```python
from build123d import *

# Parameters (mm, degrees)
F0_W     = 100.119468
F0_H     = 86.142674
F1_DEPTH = 50.8
F2_R     = 25.4
F4_D     = 25.4


with BuildPart() as f1:
    # F0 (on Front) → F1 (new body)
    with BuildSketch(Plane.XZ):
        with Locations((1.568822, 9.270322)):
            Rectangle(F0_W, F0_H)
    extrude(amount=F1_DEPTH)

    # F2
    f2_edges = [f1.edges().sort_by_distance(p)[0] for p in [
        (51.628556, -25.4, 52.341659),
        (-48.490912, -25.4, 52.341659),
        (-48.490912, -25.4, -33.801015),
        (51.628556, -25.4, -33.801015),
    ]]
    fillet(f2_edges, radius=F2_R)

    # F4 (through all)
    with Locations(Plane.XZ.offset(50.8)):
        with Locations((11.67061, 29.531537)):
            Hole(F4_D / 2)


solid = f1.part
```
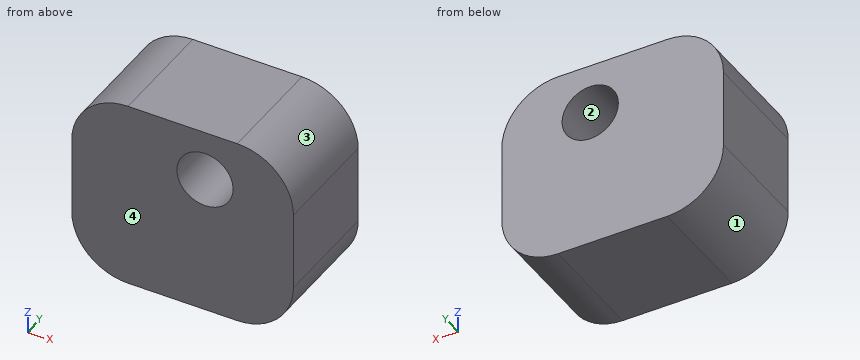
Verification items for the finished model (mm, model axes). Face numbers are marked on the shaded views. Round coordinates to 2 decimals unless told otherwise and drop trailing zeros. Write each loop counter-clockwise with the first axis right and the second up, starting at its lowest first coordinate (ties: lowest second). Pieces come first, ordered by that corner, then holes. Notation, with made-up numbers: (14.25, 12.25) - (47.25, 12.25) arc R20 cw to (47.25, 22.25) - close; hole circle Ø6 at (14, 17.5). An arc over 180 degrees is marked (long way). Answer as a JSON object with one key per item and string values. Group by question number.
Q1. Thickness scan on line 1 (Z direction, x = 12, y = -26.5); line 2 (X direction, y = -27.5, z = 35.5); line 3 (X direction, y = -29, z = 23.5). Record the ranges inside material, lowest first.
Q2. Section check D-D, the plane x = -34. Enter the section's corners in (y, z), plus the area to 3 significant figures.
Q3. Go/stop test with flat-tipped pins: pin 1 Ø2 at (y, z) = (-14, 35.5) entering from -X; pin 2 Ø8 at (x, y) = (-34, -11.5) entering from +Z; pin 3 Ø1 at (y, z) = (-43, -25) entering from -X. Record where each tip stops, or that it passes through.
Q4. Section check A-A, the plane x = 17. Enter the section's corners in (y, z), plus the area to 3 significant figures.
Q5. Section check B-B, the plane z = 31. Enter the section's corners in (x, y), plus the area to 3 significant figures.
Q6. Section check C-C, the plane y = -9.5. Enter the section's corners in (x, z), plus the area to 3 significant figures.
Q7. Mould release check, pull along Z, two halves, no side actions. Record for the marked faces 1, 2, 3 and 4: released by +Z, released by -Z, zero draft, split by the parting line, or undercut.
Found:
{
 "1": {"line 1": "z = -33.8 to 16.84, 42.23 to 52.34", "line 2": "x = -47.01 to 0.46, 22.88 to 50.14", "line 3": "x = -48.49 to 0.49, 22.85 to 51.63"},
 "2": {"outline": "(-50.8, -31.34) - (0, -31.34) - (0, 49.88) - (-50.8, 49.88) - close", "area": "4,130 mm^2"},
 "3": {"pin 1": "stops at x = -47.34", "pin 2": "stops at z = 51.38", "pin 3": "stops at x = -42.74"},
 "4": {"outline": "(-50.8, -33.8) - (0, -33.8) - (0, 18) - (-50.8, 18) - close; (-50.8, 41.06) - (0, 41.06) - (0, 52.34) - (-50.8, 52.34) - close", "area": "3,200 mm^2"},
 "5": {"outline": "(-48.16, -50.8) - (-0.94, -50.8) - (-0.94, 0) - (-48.16, 0) - close; (24.29, -50.8) - (51.3, -50.8) - (51.3, 0) - (24.29, 0) - close", "area": "3,770 mm^2"},
 "6": {"outline": "(-48.49, -8.4) arc R25.4 ccw to (-23.09, -33.8) - (26.23, -33.8) arc R25.4 ccw to (51.63, -8.4) - (51.63, 26.94) arc R25.4 ccw to (26.23, 52.34) - (-23.09, 52.34) arc R25.4 ccw to (-48.49, 26.94) - close; hole circle Ø25.4 at (11.67, 29.53)", "area": "7,560 mm^2"},
 "7": {"face 1": "released by -Z", "face 2": "undercut", "face 3": "released by +Z", "face 4": "zero draft"}
}
